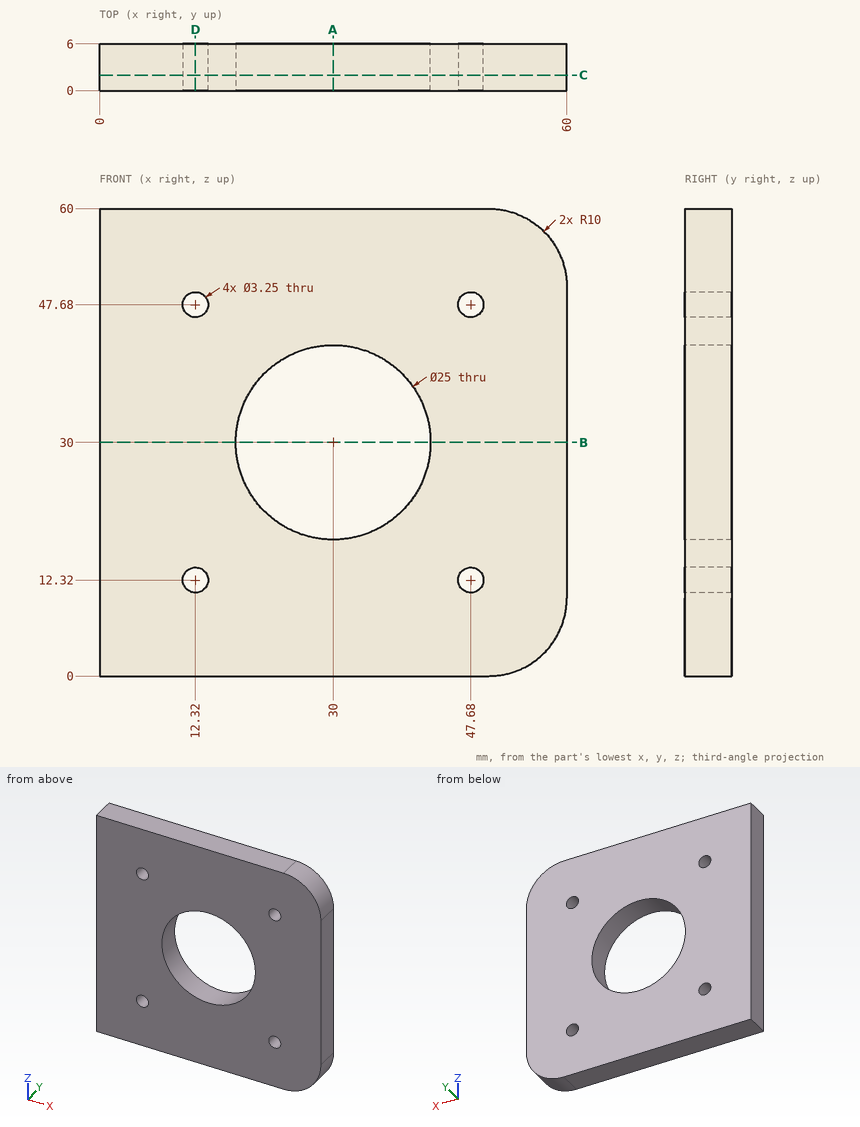
Could you check a few things on this drawing? It's one solid part, dimensions in mm from its lowest x, y, z. Coordinates: 2 decimals unless noted, no trailing zeros. Order: outer loops, then holes, each group sorted by start corner. A loop starts at its lowest first (then second) coordinate and runs counter-clockwise, first axis right, second up.
1) I need wall thicknesses on line 1 (X direction, y = 1.65, z = 47.68) (3 decimals); line 2 (X direction, y = 4.3, z = 30). Which ranges of each line are inside material? Lowest first, please.
2) Imagine slicing it at C-C on y = 2. List the corners of the cut face in (x, z) for me (3 decimals), and give its area (3 significant figures).
3) Will this pin go through, and if not, where does the flat tip stop? pin 1 (2.5 mm diameter, centred on x = 12.32, z = 12.32, fed in from +Y).
4) Imagine slicing it at B-B on z = 30. List the corners of the cut face in (x, y) for me.
5) Imagine slicing it at A-A on x = 30. List the corners of the cut face in (y, z) for me.
6) Imagine slicing it at D-D on x = 12.32. List the corners of the cut face in (y, z) for me (3 decimals).
Response values:
1. line 1: x = 0 to 10.695, 13.945 to 46.055, 49.305 to 60
1. line 2: x = 0 to 17.5, 42.5 to 60
2. outline: (0, 0) - (50, 0) arc R10 ccw to (60, 10) - (60, 50) arc R10 ccw to (50, 60) - (0, 60) - close; hole circle Ø3.25 at (12.32, 12.32); hole circle Ø3.25 at (12.32, 47.68); hole circle Ø25 at (30, 30); hole circle Ø3.25 at (47.68, 12.32); hole circle Ø3.25 at (47.68, 47.68)
2. area: 3,030 mm2
3. pin 1: passes through
4. outline: (0, 0) - (17.5, 0) - (17.5, 6) - (0, 6) - close; (42.5, 0) - (60, 0) - (60, 6) - (42.5, 6) - close
5. outline: (0, 0) - (6, 0) - (6, 17.5) - (0, 17.5) - close; (0, 42.5) - (6, 42.5) - (6, 60) - (0, 60) - close
6. outline: (0, 0) - (6, 0) - (6, 10.695) - (0, 10.695) - close; (0, 13.945) - (6, 13.945) - (6, 46.055) - (0, 46.055) - close; (0, 49.305) - (6, 49.305) - (6, 60) - (0, 60) - close
